from build123d import *

# Parameters (mm, degrees)
BLANKSKE_W         = 100
BLANKSKE_H         = 16
BLANK_DEPTH        = 15
TOOTHCUTSIM_DEPTH  = 103.376755174
TEETHCUTS_COUNT    = 33
TEETHCUTS_PITCH    = 3.14159265
SKETCH1_R          = 3.2
CUT_EXTRUDE1_DEPTH = 50
SKETCH2_W          = 40.39626908
SKETCH2_H          = 26.250089156
CUT_EXTRUDE2_DEPTH = 103.376755174


with BuildPart() as part:
    # BlankSke → Blank (new body)
    with BuildSketch(Plane.XY):
        with Locations((50, 8)):
            Rectangle(BLANKSKE_W, BLANKSKE_H)
    extrude(amount=-BLANK_DEPTH)

    # TooCutSkeSim → ToothCutSim (cut, through all)
    with BuildSketch(Plane.XY):
        Polygon((0.44443537, 13.75), (-0.44443537, 13.75), (-1.272613241, 16.0254), (1.272613241, 16.0254), align=None)
    toothcutsim = extrude(amount=-TOOTHCUTSIM_DEPTH, mode=Mode.SUBTRACT)

    # TeethCuts: ToothCutSim ×33
    with Locations(*[(i * TEETHCUTS_PITCH, 0, 0) for i in range(1, TEETHCUTS_COUNT)]):
        add(toothcutsim, mode=Mode.SUBTRACT)

    # Sketch1 → Cut-Extrude1 (cut)
    with BuildSketch(Plane(origin=(100, 0, 0), x_dir=(0, 0, -1), z_dir=(1, 0, 0))):
        with Locations(Location((7.5, 6.993868828, 0), (0, 0, 90))):
            Circle(SKETCH1_R)
    extrude(amount=-CUT_EXTRUDE1_DEPTH, mode=Mode.SUBTRACT)

    # Sketch2 → Cut-Extrude2 (cut, through all)
    with BuildSketch(Plane.XY):
        with Locations((20.19813454, 13.125044578)):
            Rectangle(SKETCH2_W, SKETCH2_H)
    extrude(amount=-CUT_EXTRUDE2_DEPTH, mode=Mode.SUBTRACT)


solid = part.part
Part model, mm, in its own coordinate system. A direction names the side the tool comes from. Round coordinates to 2 decimals unless told otherwise and drop trailing zeros. Write each loop counter-clockwise with the first axis right and the second up, starting at its lowest first coordinate (ties: lowest second). Pieces come first, ordered by that corner, then holes. Notation, with made-up numbers: M -21,49 L -1,49 A6 cw -1,60 Z; hole C -7.5,-13 d11. An arc over 180 degrees is marked long. Return JSON: item names as keys, results as strings. Group by question number.
(1) Drill centre lines: probe 1 along Z at (x, y) = (87.5, 9.5); probe 2 along X at (y, z) = (7, -7); probe 3 along Y at (x, z) = (69.5, -10). Where is each one in solid material? Low to high.
(2) Saw through at A-A on y = 5.25. Write the cut outline in (x, z), then the cut area to 3 significant figures.
(3) Pin check, flat tip, straight feed: pin 1 Ø0.7 at (x, z) = (66, -6.5) entering from +Y. Stop position of the tip, or through.
(4) Which spindle directions (+Z, -Z, +X, -X, +Y, -Y) get a long thin tool onto all of the face, cutting with end or side? Do faces 4 (the face through (90.258, 14.859, -7.395)), 5 (the face through (70, 0, -7)), 6 (the face through (75.35, 6.577, -4.327)). Say none if no direction does.
(5) Saw through at B-B on y = 15. Count the separate pieces of the cut face and the enclosed holes in it, then the cut area to 3 significant figures.
(6) Two-plate mould, pull along X, no slides. Class faces 1 (the face through (70, 8, -15)), 2 (the face through (100, 7, -11)), 3 (the face through (80.833, 14.859, -7.395)): +X half, -X half, draft (parallel to the pull), parting line (faces both ways), or undercut.
Returned:
{
 "1": {"probe 1": "-15 to -9.49, -5.51 to 0", "probe 2": "40.4 to 50", "probe 3": "0 to 5, 8.99 to 13.75"},
 "2": {"outline": "M 40.4,-15 L 100,-15 L 100,-10.18 L 50,-10.18 L 50,-4.82 L 100,-4.82 L 100,0 L 40.4,0 Z", "area": "626 mm²"},
 "3": {"pin 1": "y = 13.75"},
 "4": {"face 4": "+Z, -Z, +Y", "face 5": "+Z, -Z, +X, -X, -Y", "face 6": "+X"},
 "5": {"separate pieces": "19", "enclosed holes": "0", "area": "383 mm²"},
 "6": {"face 1": "draft", "face 2": "+X half", "face 3": "undercut"}
}
